Geometry: final body of the model. Coordinates: model frame, mm. Face numbers are marked on the shaded views. A direction names the side the tool comes from. Give positions to 0.01 mm unless a question says otherwise; leave off trailing zeros. Order: outer loops, then holes, each group sorted by start corner. A loop starts at its lowest first (then second) coordinate and runs counter-clockwise, first axis right, second up. Notation, with made-up numbers: (54.5, 86) - (71.5, 86) arc R21 ccw to (71.5, 122) - close; hole circle Ø1 at (43.5, 87.5). An arc over 180 degrees is marked (long way). Use one line per item in the form item = value.
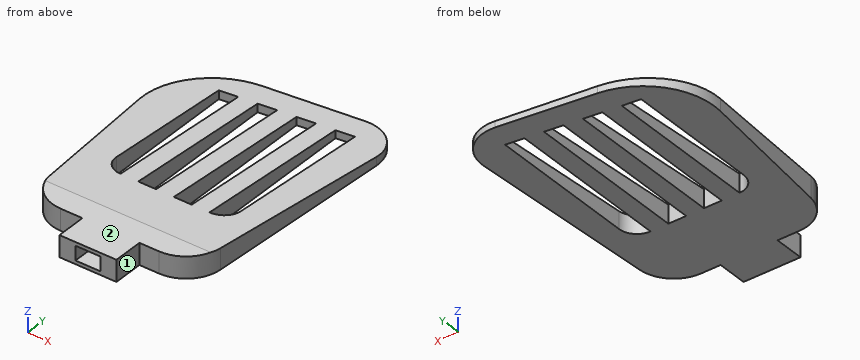
from build123d import *

# Parameters (mm, degrees)
F1_DEPTH      = 6
F3_DEPTH      = 32.218832
F3_DEPTH_BACK = 22.944034
F4_W          = 7
F4_H          = 4
F5_DEPTH      = 9


with BuildPart() as f1:
    # F0 (on Top) → F1 (new body)
    with BuildSketch(Plane.XY):
        with BuildLine():
            Line((-1.988453, 8.411565), (-1.988453, 0))
            Line((-1.988453, 0), (14.011547, 0))
            Line((14.011547, 0), (14.011547, 8.411565))
            Line((14.011547, 8.411565), (19.504514, 8.411565))
            ThreePointArc((19.504514, 8.411565), (26.394687, 11.164117), (29.491749, 17.906464))
            Line((29.491749, 17.906464), (32.205068, 71.556178))
            ThreePointArc((32.205068, 71.556178), (29.038679, 79.374011), (21.019631, 81.989235))
            Line((21.019631, 81.989235), (-5.339437, 78.807969))
            ThreePointArc((-5.339437, 78.807969), (-18.677797, 71.297794), (-22.798946, 56.555653))
            Line((-22.798946, 56.555653), (-18.050739, 17.213364))
            ThreePointArc((-18.050739, 17.213364), (-14.75671, 10.928852), (-8.122783, 8.411565))
            Line((-8.122783, 8.411565), (-1.988453, 8.411565))
        make_face()
        with BuildLine():
            Line((-11.620977, 33.411565), (-11.620977, 70.999055))
            Line((-11.620977, 70.999055), (-6.620977, 71.602503))
            Line((-6.620977, 71.602503), (-6.620977, 28.411565))
            ThreePointArc((-6.620977, 28.411565), (-10.15651, 29.876032), (-11.620977, 33.411565))
        make_face(mode=Mode.SUBTRACT)
        Polygon((-1.620977, 28.411565), (-1.620977, 72.205952), (3.379023, 72.8094), (3.379023, 28.411565), align=None, mode=Mode.SUBTRACT)
        Polygon((8.379023, 73.412848), (13.379023, 74.016297), (13.379023, 28.411565), (8.379023, 28.411565), align=None, mode=Mode.SUBTRACT)
        with BuildLine():
            Line((23.379023, 75.223193), (23.379023, 33.411565))
            ThreePointArc((23.379023, 33.411565), (21.914557, 29.876032), (18.379023, 28.411565))
            Line((18.379023, 28.411565), (18.379023, 74.619745))
            Line((18.379023, 74.619745), (23.379023, 75.223193))
        make_face(mode=Mode.SUBTRACT)
    extrude(amount=F1_DEPTH)

    # F2 (on Right) → F3 (cut, two sides)
    with BuildSketch(Plane.YZ) as f3_sk:
        Polygon((82.888745, 7.075289), (8.152761, 6.443492), (82.888745, 1.665537), align=None)
    extrude(amount=F3_DEPTH, mode=Mode.SUBTRACT)
    extrude(f3_sk.sketch, amount=-F3_DEPTH_BACK, mode=Mode.SUBTRACT)

    # F4 (on face) → F5 (cut)
    with BuildSketch(Plane.XZ):
        with Locations((6.011547, 3)):
            Rectangle(F4_W, F4_H)
    extrude(amount=-F5_DEPTH, mode=Mode.SUBTRACT)


solid = f1.part
(1) Cut plane B-B on x = 10.5. Output: boundary loops of the cut face in (y, z), plus the area to 3 significant figures.
Computed values:
outline = (0, 0) - (28.41, 0) - (28.41, 5.15) - (15.09, 6) - (0, 6) - close; (73.67, 0) - (80.72, 0) - (80.72, 1.8) - (73.67, 2.25) - close
area = 179 mm²
(2) Contact query for flat-ended pins moving along their axis: pin 1 Ø1 at (x, z) = (-6, 5) entering from -Y; pin 2 Ø1.5 at (x, z) = (11.5, 1.5) entering from +Y; pin 3 Ø1.4 at (y, z) = (60.5, 2) entering from +X. Output: stop coordinate, or through.
Computed values:
pin_1 = 8.41
pin_2 = 80.93
pin_3 = 31.68
(3) Ray query, line 1 along X through (y, z) = (8, 1.5); line 2 along X through (y, z) = (54, 2.5); line 3 along X through (y, z) = (36, 1.5). Return the intervals inside material, ascending.
Computed values:
line_1 = -1.99 to 2.51, 9.51 to 14.01
line_2 = -22.49 to -11.62, -6.62 to -1.62, 3.38 to 8.38, 13.38 to 18.38, 23.38 to 31.32
line_3 = -20.32 to -11.62, -6.62 to -1.62, 3.38 to 8.38, 13.38 to 18.38, 23.38 to 30.41
(4) Cut plane D-D on x = 25. Output: boundary loops of the cut face in (y, z), plus the area to 3 significant figures.
Computed values:
outline = (10.06, 0) - (81.67, 0) - (81.67, 1.74) - (15.09, 6) - (10.06, 6) - close
area = 288 mm²
(5) Reachability of the marked faces 1 and 2 from +Z, -Z, +X, -X, +Y, -Y: full face, straight path, thin tool, end or side. Return the list, or none.
Computed values:
face_1 = +Z, -Z, +X, -Y
face_2 = +Z, +X, -X, +Y, -Y
(6) Cut plane C-C on y = 32.5. Output: boundary loops of the cut face in (x, z), plus the area to 3 significant figures.
Computed values:
outline = (-19.9, 0) - (-11.54, 0) - (-11.54, 4.89) - (-19.9, 4.89) - close; (-6.62, 0) - (-1.62, 0) - (-1.62, 4.89) - (-6.62, 4.89) - close; (3.38, 0) - (8.38, 0) - (8.38, 4.89) - (3.38, 4.89) - close; (13.38, 0) - (18.38, 0) - (18.38, 4.89) - (13.38, 4.89) - close; (23.3, 0) - (30.23, 0) - (30.23, 4.89) - (23.3, 4.89) - close
area = 148 mm²
(7) Cut plane A-A on y = 54.5. Output: boundary loops of the cut face in (x, z).
Computed values:
outline = (-22.55, 0) - (-11.62, 0) - (-11.62, 3.48) - (-22.55, 3.48) - close; (-6.62, 0) - (-1.62, 0) - (-1.62, 3.48) - (-6.62, 3.48) - close; (3.38, 0) - (8.38, 0) - (8.38, 3.48) - (3.38, 3.48) - close; (13.38, 0) - (18.38, 0) - (18.38, 3.48) - (13.38, 3.48) - close; (23.38, 0) - (31.34, 0) - (31.34, 3.48) - (23.38, 3.48) - close
